Source: CAD feature listing. Evaluate the final solid. Frame: model axes, mm. A direction names the side the tool comes from. Coordinates: 2 decimals unless noted, no trailing zeros. Order: outer loops, then holes, each group sorted by start corner. A loop starts at its lowest first (then second) coordinate and runs counter-clockwise, first axis right, second up. Notation, with made-up numbers: (88, 53.5) -> (118, 53.5) arc R11 cw to (118, 60.5) -> close; hole circle Ø10 at (84, 89.5). An arc over 180 degrees is marked (long way). Write item = value, one per line. Start each with the question number.
Item 1: Set-up query: faces 5 (the cylindrical face through (33.1, -14.64, -15.78)), 6 (the cylindrical face through (-33.14, -14.6, -15.78)), 7 (the cylindrical face through (29.21, 0.9, -6.08)), 8 (the flat face through (-25, -2, 1)). Return all of +Z, -Z, +X, -X, +Y, -Y with unobstructed straight access to the full face (end or side cutting, diameter ignored); none if empty.
Item 2: Section query B-B (x = 26.35). Output: boundary loops of the cut face in (y, z), then the cut area to 3 significant figures.
Item 3: Contact query for flat-ended pins moving along their axis: pin 1 (1 mm diameter, centred on y = 0.5, z = -19.5, fed in from +X); pin 2 (0.9 mm diameter, centred on y = 13.5, z = -26, fed in from +X); pin 3 (4 mm diameter, centred on x = 38.5, z = 0.5, fed in from -Y). Output: stop coordinate, or through.
Item 4: Section query C-C (x = -16). Output: boundary loops of the cut face in (y, z).
Item 5: Section query A-A (z = -1.5). Output: boundary loops of the cut face in (x, y), then the cut area to 3 significant figures.
Item 6: Section query D-D (z = -28.5). Output: boundary loops of the cut face in (x, y).
Item 7: Mould query, pull axis Y, two halves, no side actions, for faces 1 (the flat face through (-41.4, -10.32, 1.97)), 2 (the flat face through (1, 0, 4)), 3 (the cylindrical face through (38, 0, 2)), 4 (the cylindrical face through (-33.1, 14.64, -15.78)). Classes: released by +Y, released by -Y, zero draft, split by the parting line, or undercut.
Item 8: Ray query, line 1 along Y through (x, z) = (13, 2); line 2 along Y through (x, z) = (23.5, -19); line 3 along X through (y, z) = (-5, -8). Return the intervals inside material, ascending. Write a range as [from, to].
```python
from build123d import *

# Parameters (mm, degrees)
CROQUIS1_R                 = 2
CROQUIS1_R_2               = 3.5
CROQUIS1_R_3               = 9
SALIENTE_EXTRUIR1_DEPTH    = 4
SALIENTE_EXTRUIR2_START    = -12
CROQUIS3_R                 = 3
CROQUIS3_R_2               = 2
SALIENTE_EXTRUIR2_DEPTH    = 12
CROQUIS4_W                 = 62
CROQUIS4_H                 = 25
SALIENTE_EXTRUIR3_DEPTH    = 32
CORTAR_EXTRUIR1_DEPTH      = 10
CORTAR_EXTRUIR1_DEPTH_BACK = 18
CROQUIS5_R                 = 4.5
CROQUIS5_W                 = 17.5
CROQUIS5_H                 = 18.482527597
CORTAR_EXTRUIR2_START      = -3
CROQUIS6_R                 = 4
CROQUIS6_R_2               = 2
CORTAR_EXTRUIR2_DEPTH      = 3


with BuildPart() as part:
    # Croquis1 → Saliente-Extruir1 (new body)
    with BuildSketch(Plane.XY):
        Polygon((-34, 15.5), (34, 15.5), (49, 5), (49, -5), (34, -15.5), (-34, -15.5), (-49, -5), (-49, 5), align=None)
        with Locations((-26.35, 0)):
            Circle(CROQUIS1_R, mode=Mode.SUBTRACT)
        with Locations((26.35, 0)):
            Circle(CROQUIS1_R, mode=Mode.SUBTRACT)
        with Locations((-41.5, 0)):
            Circle(CROQUIS1_R_2, mode=Mode.SUBTRACT)
        with Locations((41.5, 0)):
            Circle(CROQUIS1_R_2, mode=Mode.SUBTRACT)
        with Locations((-13, 3)):
            Circle(CROQUIS1_R_3, mode=Mode.SUBTRACT)
        with Locations((13, 3)):
            Circle(CROQUIS1_R_3, mode=Mode.SUBTRACT)
    extrude(amount=SALIENTE_EXTRUIR1_DEPTH)

    # Croquis3 → Saliente-Extruir2 (add)
    # profile 1 of 2: a face of its own
    with BuildSketch(Plane.XY.offset(SALIENTE_EXTRUIR2_START)):
        with Locations((26.35, 0)):
            Circle(CROQUIS3_R)
        with Locations((26.35, 0)):
            Circle(CROQUIS3_R_2, mode=Mode.SUBTRACT)
    # profile 2 of 2: a face of its own
    with BuildSketch(Plane.XY.offset(SALIENTE_EXTRUIR2_START)):
        with Locations((-26.35, 0)):
            Circle(CROQUIS3_R)
        with Locations((-26.35, 0)):
            Circle(CROQUIS3_R_2, mode=Mode.SUBTRACT)
    extrude(amount=SALIENTE_EXTRUIR2_DEPTH)

    # Croquis4 → Saliente-Extruir3 (add)
    with BuildSketch(Plane.XY):
        with BuildLine():
            Line((31, 15.5), (-31, 15.5))
            ThreePointArc((-31, 15.5), (-33.121320344, 14.621320344), (-34, 12.5))
            Line((-34, 12.5), (-34, -12.5))
            ThreePointArc((-34, -12.5), (-33.121320344, -14.621320344), (-31, -15.5))
            Line((-31, -15.5), (31, -15.5))
            ThreePointArc((31, -15.5), (33.121320344, -14.621320344), (34, -12.5))
            Line((34, -12.5), (34, 12.5))
            ThreePointArc((34, 12.5), (33.121320344, 14.621320344), (31, 15.5))
        make_face()
        Rectangle(CROQUIS4_W, CROQUIS4_H, mode=Mode.SUBTRACT)
    extrude(amount=-SALIENTE_EXTRUIR3_DEPTH)

    # Croquis5 → Cortar-Extruir1 (cut, two sides: drawn at the far end of the back side and taken through both)
    with BuildSketch(Plane(origin=(0, 16, 0), x_dir=(1, 0, 0), z_dir=(0, 1, 0)).offset(-CORTAR_EXTRUIR1_DEPTH_BACK)):
        with Locations((-18.75, 22.773683321)):
            Circle(CROQUIS5_R)
        with Locations((0, 22.77368332)):
            Rectangle(CROQUIS5_W, CROQUIS5_H)
    extrude(amount=CORTAR_EXTRUIR1_DEPTH + CORTAR_EXTRUIR1_DEPTH_BACK, mode=Mode.SUBTRACT)

    # Croquis6 → Cortar-Extruir2 (cut)
    # profile 1 of 2: a face of its own
    with BuildSketch(Plane.XY.offset(4).offset(CORTAR_EXTRUIR2_START)):
        with Locations((26.35, 0)):
            Circle(CROQUIS6_R)
        with Locations((26.35, 0)):
            Circle(CROQUIS6_R_2, mode=Mode.SUBTRACT)
    # profile 2 of 2: a face of its own
    with BuildSketch(Plane.XY.offset(4).offset(CORTAR_EXTRUIR2_START)):
        with Locations((-26.35, 0)):
            Circle(CROQUIS6_R)
        with Locations((-26.35, 0)):
            Circle(CROQUIS6_R_2, mode=Mode.SUBTRACT)
    extrude(amount=CORTAR_EXTRUIR2_DEPTH, mode=Mode.SUBTRACT)


solid = part.part
```
Computed:
q1.face_5 = -Z, +X, -Y
q1.face_6 = -Z, -X, -Y
q1.face_7 = -Z
q1.face_8 = +Z
q2.outline = (-15.5, -32) -> (-12.5, -32) -> (-12.5, 0) -> (-3, 0) -> (-3, -12) -> (-2, -12) -> (-2, 1) -> (-4, 1) -> (-4, 4) -> (-15.5, 4) -> close; (2, -12) -> (3, -12) -> (3, 0) -> (12.5, 0) -> (12.5, -32) -> (15.5, -32) -> (15.5, 4) -> (4, 4) -> (4, 1) -> (2, 1) -> close
q2.area = 312 mm^2
q3.pin_1 = 34
q3.pin_2 = 33.95
q3.pin_3 = -13.75
q4.outline = (-15.5, -32) -> (-12.5, -32) -> (-12.5, 0) -> (-5.49, 0) -> (-5.49, 4) -> (-15.5, 4) -> close; (11.49, 0) -> (12.5, 0) -> (12.5, -19.21) -> (15.5, -19.21) -> (15.5, 4) -> (11.49, 4) -> close; (12.5, -32) -> (15.5, -32) -> (15.5, -26.34) -> (12.5, -26.34) -> close
q5.outline = (-34, -12.5) arc R3 ccw to (-31, -15.5) -> (31, -15.5) arc R3 ccw to (34, -12.5) -> (34, 12.5) arc R3 ccw to (31, 15.5) -> (-31, 15.5) arc R3 ccw to (-34, 12.5) -> close; circle Ø6 at (-26.35, 0); circle Ø6 at (26.35, 0); hole (-31, -12.5) -> (31, -12.5) -> (31, 12.5) -> (-31, 12.5) -> close; hole circle Ø4 at (-26.35, 0); hole circle Ø4 at (26.35, 0)
q5.area = 582 mm^2
q6.outline = (-34, -12.5) arc R3 ccw to (-31, -15.5) -> (31, -15.5) arc R3 ccw to (34, -12.5) -> (34, 12.5) arc R3 ccw to (31, 15.5) -> (8.75, 15.5) -> (8.75, 12.5) -> (31, 12.5) -> (31, -12.5) -> (-31, -12.5) -> (-31, 12.5) -> (-8.75, 12.5) -> (-8.75, 15.5) -> (-31, 15.5) arc R3 ccw to (-34, 12.5) -> close
q7.face_1 = released by -Y
q7.face_2 = zero draft
q7.face_3 = undercut
q7.face_4 = released by +Y
q8.line_1 = [-15.5, -6], [12, 15.5]
q8.line_2 = [-15.5, -12.5], [12.5, 15.5]
q8.line_3 = [-34, -31], [31, 34]
